Verification items for the finished model (mm, model axes). Give positions to 0.01 mm unless a question says otherwise; leave off trailing zeros. Order: outer loops, then holes, each group sorted by start corner. A loop starts at its lowest first (then second) coordinate and runs counter-clockwise, first axis right, second up. Notation, with made-up numbers: (68, 27.5) -> (100, 27.5) arc R32 ccw to (100, 57.5) -> close; hole circle Ø8 at (41.25, 80). An arc over 180 degrees is marked (long way). Write each question's results on one line, items separated by ' | '. Start each with the question number.
1. Cross-section at A-A, the plane y = -45. Enter the section's corners in (x, z), then the cut area to 3 significant figures.
2. Material ranges on L1, parallel to Y at x = 7.75, z = 3; L2, parallel to Z at x = 10, y = 45; L3, parallel to X at y = 43, z = 1.75, recorded low to high. Write a range as from..to.
3. Depth check by flat-ended pin: pin 1 Ø2.5 at (y, z) = (-45, 3) entering from -X. Enter the tip coordinate at first touch or a pass-through.
4. Cross-section at B-B, the plane z = 3. Enter the section's corners in (x, y).
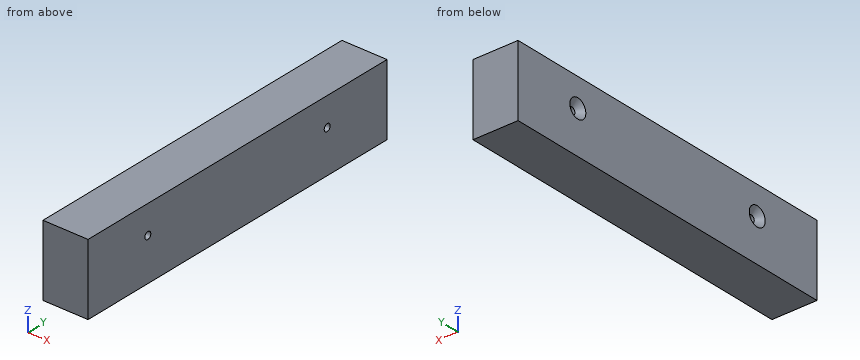
from build123d import *

# Parameters (mm, degrees)
F2_W           = 19
F2_H           = 30
F3_DEPTH       = 75
F5_D           = 3
F5_CSINK_D     = 8
F5_CSINK_ANGLE = 90


with BuildPart() as f3:
    # F2 (on Front) → F3 (new body, symmetric)
    with BuildSketch(Plane.XZ):
        with Locations((9.5, 0)):
            Rectangle(F2_W, F2_H)
    extrude(amount=F3_DEPTH, both=True)

    # F5 (through all)
    with Locations(Plane(origin=(0, 0, 0), x_dir=(0, -1, 0), z_dir=(-1, 0, 0))):
        with Locations((-45, 3), (45, 3)):
            CounterSinkHole(F5_D / 2, F5_CSINK_D / 2, counter_sink_angle=F5_CSINK_ANGLE)


solid = f3.part
Results below:
1) outline: (0, -15) -> (19, -15) -> (19, 1.5) -> (2.5, 1.5) -> (0, -1) -> close; (0, 7) -> (2.5, 4.5) -> (19, 4.5) -> (19, 15) -> (0, 15) -> close | area: 507 mm²
2) L1: y = -75..-46.5, -43.5..43.5, 46.5..75 | L2: z = -15..1.5, 4.5..15 | L3: x = 1.64..19
3) pin 1: passes through
4) outline: (0, -75) -> (19, -75) -> (19, -46.5) -> (2.5, -46.5) -> (0, -49) -> close; (0, -41) -> (2.5, -43.5) -> (19, -43.5) -> (19, 43.5) -> (2.5, 43.5) -> (0, 41) -> close; (0, 49) -> (2.5, 46.5) -> (19, 46.5) -> (19, 75) -> (0, 75) -> close
